from build123d import *

# Parameters (mm, degrees)
F0_W     = 16.1
F0_H     = 6
F1_DEPTH = 11.3
F2_DEPTH = 6
F3_DEPTH = 10


with BuildPart() as f1:
    # F0 (on Top) → F1 (new body)
    with BuildSketch(Plane.XY):
        with BuildLine():
            Line((59.8, 7.4), (3.7, 7.4))
            ThreePointArc((3.7, 7.4), (4.837981, 7.220653), (5.865641, 6.7))
            Line((5.865641, 6.7), (23.7, 6.7))
            Line((23.7, 6.7), (39.8, 6.7))
            Line((39.8, 6.7), (57.634359, 6.7))
            ThreePointArc((57.634359, 6.7), (58.662019, 7.220653), (59.8, 7.4))
        make_face()
        with BuildLine():
            ThreePointArc((57.634359, 6.7), (56.1, 3.7), (57.634359, 0.7))
            Line((57.634359, 0.7), (59.8, 0.7))
            ThreePointArc((59.8, 0.7), (56.8, 3.7), (59.8, 6.7))
            Line((59.8, 6.7), (57.634359, 6.7))
        make_face()
        with BuildLine():
            ThreePointArc((59.8, 7.4), (62.416295, 6.316295), (63.5, 3.7))
            Line((63.5, 3.7), (63.5, 7.4))
            Line((63.5, 7.4), (59.8, 7.4))
        make_face()
        with BuildLine():
            ThreePointArc((63.5, 3.7), (62.416295, 1.083705), (59.8, 0))
            Line((59.8, 0), (63.5, 0))
            Line((63.5, 0), (63.5, 3.7))
        make_face()
        with BuildLine():
            ThreePointArc((5.865641, 0.7), (4.837981, 0.179347), (3.7, 0))
            Line((3.7, 0), (59.8, 0))
            ThreePointArc((59.8, 0), (58.662019, 0.179347), (57.634359, 0.7))
            Line((57.634359, 0.7), (39.8, 0.7))
            Line((39.8, 0.7), (23.7, 0.7))
            Line((23.7, 0.7), (5.865641, 0.7))
        make_face()
        with BuildLine():
            ThreePointArc((57.634359, 0.7), (58.662019, 0.179347), (59.8, 0))
            ThreePointArc((59.8, 0), (62.416295, 1.083705), (63.5, 3.7))
            ThreePointArc((63.5, 3.7), (62.416295, 6.316295), (59.8, 7.4))
            ThreePointArc((59.8, 7.4), (58.662019, 7.220653), (57.634359, 6.7))
            Line((57.634359, 6.7), (59.8, 6.7))
            ThreePointArc((59.8, 6.7), (61.92132, 5.82132), (62.8, 3.7))
            ThreePointArc((62.8, 3.7), (61.92132, 1.57868), (59.8, 0.7))
            Line((59.8, 0.7), (57.634359, 0.7))
        make_face()
        with Locations((31.75, 3.7)):
            Rectangle(F0_W, F0_H)
        with BuildLine():
            ThreePointArc((0, 3.7), (1.083705, 1.083705), (3.7, 0))
            ThreePointArc((3.7, 0), (4.837981, 0.179347), (5.865641, 0.7))
            Line((5.865641, 0.7), (3.7, 0.7))
            ThreePointArc((3.7, 0.7), (0.7, 3.7), (3.7, 6.7))
            Line((3.7, 6.7), (5.865641, 6.7))
            ThreePointArc((5.865641, 6.7), (4.837981, 7.220653), (3.7, 7.4))
            ThreePointArc((3.7, 7.4), (1.083705, 6.316295), (0, 3.7))
        make_face()
        with BuildLine():
            Line((3.7, 0.7), (5.865641, 0.7))
            ThreePointArc((5.865641, 0.7), (6.994152, 2.015196), (7.4, 3.7))
            ThreePointArc((7.4, 3.7), (6.994152, 5.384804), (5.865641, 6.7))
            Line((5.865641, 6.7), (3.7, 6.7))
            ThreePointArc((3.7, 6.7), (5.82132, 5.82132), (6.7, 3.7))
            ThreePointArc((6.7, 3.7), (5.82132, 1.57868), (3.7, 0.7))
        make_face()
        with BuildLine():
            Line((0, 7.4), (0, 3.7))
            ThreePointArc((0, 3.7), (1.083705, 6.316295), (3.7, 7.4))
            Line((3.7, 7.4), (0, 7.4))
        make_face()
        with BuildLine():
            Line((0, 3.7), (0, 0))
            Line((0, 0), (3.7, 0))
            ThreePointArc((3.7, 0), (1.083705, 1.083705), (0, 3.7))
        make_face()
        with BuildLine():
            ThreePointArc((3.7, 6.7), (0.7, 3.7), (3.7, 0.7))
            ThreePointArc((3.7, 0.7), (5.82132, 1.57868), (6.7, 3.7))
            ThreePointArc((6.7, 3.7), (5.82132, 5.82132), (3.7, 6.7))
        make_face()
        with BuildLine():
            ThreePointArc((7.4, 3.7), (6.994152, 2.015196), (5.865641, 0.7))
            Line((5.865641, 0.7), (23.7, 0.7))
            Line((23.7, 0.7), (23.7, 6.7))
            Line((23.7, 6.7), (5.865641, 6.7))
            ThreePointArc((5.865641, 6.7), (6.994152, 5.384804), (7.4, 3.7))
        make_face()
        with BuildLine():
            Line((39.8, 0.7), (57.634359, 0.7))
            ThreePointArc((57.634359, 0.7), (56.1, 3.7), (57.634359, 6.7))
            Line((57.634359, 6.7), (39.8, 6.7))
            Line((39.8, 6.7), (39.8, 0.7))
        make_face()
        with BuildLine():
            ThreePointArc((59.8, 6.7), (56.8, 3.7), (59.8, 0.7))
            ThreePointArc((59.8, 0.7), (61.92132, 1.57868), (62.8, 3.7))
            ThreePointArc((62.8, 3.7), (61.92132, 5.82132), (59.8, 6.7))
        make_face()
    extrude(amount=-F1_DEPTH)

    # F0 (on Top) → F2 (cut)
    with BuildSketch(Plane.XY):
        with BuildLine():
            ThreePointArc((3.7, 6.7), (0.7, 3.7), (3.7, 0.7))
            ThreePointArc((3.7, 0.7), (5.82132, 1.57868), (6.7, 3.7))
            ThreePointArc((6.7, 3.7), (5.82132, 5.82132), (3.7, 6.7))
        make_face()
        with BuildLine():
            ThreePointArc((59.8, 6.7), (56.8, 3.7), (59.8, 0.7))
            ThreePointArc((59.8, 0.7), (61.92132, 1.57868), (62.8, 3.7))
            ThreePointArc((62.8, 3.7), (61.92132, 5.82132), (59.8, 6.7))
        make_face()
    extrude(amount=-F2_DEPTH, mode=Mode.SUBTRACT)

    # F0 (on Top) → F3 (cut)
    with BuildSketch(Plane.XY):
        with BuildLine():
            ThreePointArc((7.4, 3.7), (6.994152, 2.015196), (5.865641, 0.7))
            Line((5.865641, 0.7), (23.7, 0.7))
            Line((23.7, 0.7), (23.7, 6.7))
            Line((23.7, 6.7), (5.865641, 6.7))
            ThreePointArc((5.865641, 6.7), (6.994152, 5.384804), (7.4, 3.7))
        make_face()
        with BuildLine():
            Line((39.8, 0.7), (57.634359, 0.7))
            ThreePointArc((57.634359, 0.7), (56.1, 3.7), (57.634359, 6.7))
            Line((57.634359, 6.7), (39.8, 6.7))
            Line((39.8, 6.7), (39.8, 0.7))
        make_face()
    extrude(amount=-F3_DEPTH, mode=Mode.SUBTRACT)


solid = f1.part
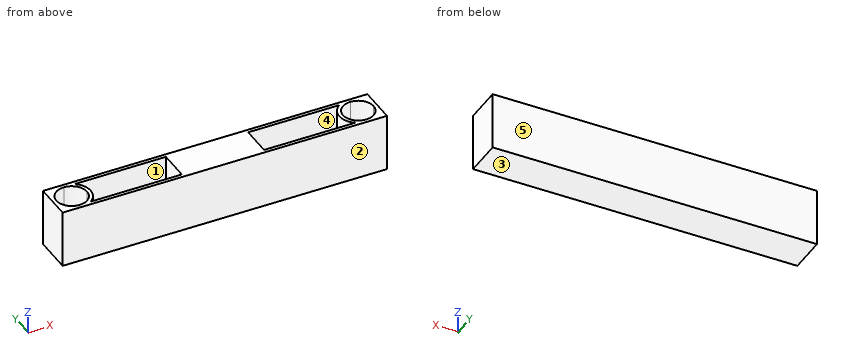
Read the model definition and answer for the solid it produces. Units are mm, in the model's axes. Face numbers are marked on the shaded views. A direction names the side the tool comes from. Round coordinates to 2 decimals unless told otherwise and drop trailing zeros. Order: outer loops, then holes, each group sorted by start corner. A loop starts at its lowest first (then second) coordinate and runs counter-clockwise, first axis right, second up. Notation, with made-up numbers: (-2.5, 26.5) - (37.5, 26.5) arc R8 ccw to (37.5, 40.5) - close; hole circle Ø10 at (85, -39). An arc over 180 degrees is marked (long way). Use one line per item in the form item = value. Start each with the question number.
(1) Find the intervals of material crossed by line 1 along X through (y, z) = (3.5, -6.75); line 2 along Y through (x, z) = (55, -7); line 3 along X through (y, z) = (1.25, -3), in increasing order. Write a range as from..to.
(2) The part is cut by section A-A (z = -2.25). Give the vertices of the cut face in (x, y).
(3) The part is cut by section C-C (y = 2.75). Give the vertices of the cut face in (x, z).
(4) For the marked faces 1 and 2, determine the directions among +Z, -Z, +X, -X, +Y, -Y from which every point of the face is accessible in a straight line to the end or side of a thin tool.
(5) The part is cut by section B-B (x = 47). Give the vertices of the cut face in (y, z).
(6) Determine the mould class of the marked faces 3, 4 and 5 for opening direction Y: +Y half, -Y half, draft (parallel to the pull), parting line (faces both ways), or undercut.
(7) A flat-ended cylindrical pin translates along its axis: pin 1 Ø1 at (x, y) = (48.5, 4.5) entering from +Z. Find the tip coordinate at first contact, or state that the pin passes through.
Checked values:
q1.line_1 = 0..7.39, 23.7..39.8, 56.11..63.5
q1.line_2 = 0..0.7, 6.7..7.4
q1.line_3 = 0..1.97, 5.43..6.47, 23.7..39.8, 57.03..58.07, 61.53..63.5
q2.outline = (0, 0) - (63.5, 0) - (63.5, 7.4) - (0, 7.4) - close; hole (3.7, 0.7) arc R3 ccw to (6.7, 3.7) arc R3 ccw to (3.7, 6.7) arc R3 ccw to start; hole (5.87, 0.7) - (23.7, 0.7) - (23.7, 6.7) - (5.87, 6.7) arc R3.7 cw to (7.4, 3.7) arc R3.7 cw to start; hole (39.8, 0.7) - (57.63, 0.7) arc R3.7 cw to (57.63, 6.7) - (39.8, 6.7) - close; hole (59.8, 0.7) arc R3 ccw to (62.8, 3.7) arc R3 ccw to (59.8, 6.7) arc R3 ccw to start
q3.outline = (0, -11.3) - (63.5, -11.3) - (63.5, 0) - (62.65, 0) - (62.65, -6) - (56.95, -6) - (56.95, 0) - (56.22, 0) - (56.22, -10) - (39.8, -10) - (39.8, 0) - (23.7, 0) - (23.7, -10) - (7.28, -10) - (7.28, 0) - (6.55, 0) - (6.55, -6) - (0.85, -6) - (0.85, 0) - (0, 0) - close
q4.face_1 = +Z
q4.face_2 = +Z, -Z, +X, -X, -Y
q5.outline = (0, -11.3) - (7.4, -11.3) - (7.4, 0) - (6.7, 0) - (6.7, -10) - (0.7, -10) - (0.7, 0) - (0, 0) - close
q6.face_3 = draft
q6.face_4 = undercut
q6.face_5 = +Y half
q7.pin_1 = -10
